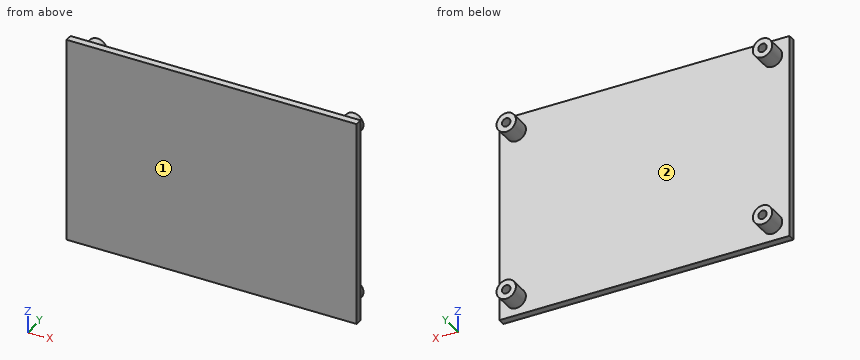
```python
from build123d import *

# Parameters (mm, degrees)
SKETCH1_W           = 120
SKETCH1_H           = 85
BOSS_EXTRUDE1_DEPTH = 3
SKETCH2_R           = 4
SKETCH2_R_2         = 1.75
BOSS_EXTRUDE2_DEPTH = 7.5


with BuildPart() as part:
    # Sketch1 → Boss-Extrude1 (new body)
    with BuildSketch(Plane(origin=(0, 0, 0), x_dir=(1, 0, 0), z_dir=(0, 1, 0))):
        with Locations((60, 42.5)):
            Rectangle(SKETCH1_W, SKETCH1_H)
    extrude(amount=BOSS_EXTRUDE1_DEPTH)

    # Sketch2 → Boss-Extrude2 (add)
    # profile 1 of 4: a face of its own
    with BuildSketch(Plane(origin=(0, 3, 0), x_dir=(1, 0, 0), z_dir=(0, 1, 0))):
        with Locations(Location((7, 78, 0), (0, 0, 90))):
            Circle(SKETCH2_R)
        with Locations(Location((7, 78, 0), (0, 0, 270))):
            Circle(SKETCH2_R_2, mode=Mode.SUBTRACT)
    # profile 2 of 4: a face of its own
    with BuildSketch(Plane(origin=(0, 3, 0), x_dir=(1, 0, 0), z_dir=(0, 1, 0))):
        with Locations(Location((7, 7, 0), (0, 0, 90))):
            Circle(SKETCH2_R)
        with Locations(Location((7, 7, 0), (0, 0, 270))):
            Circle(SKETCH2_R_2, mode=Mode.SUBTRACT)
    # profile 3 of 4: a face of its own
    with BuildSketch(Plane(origin=(0, 3, 0), x_dir=(1, 0, 0), z_dir=(0, 1, 0))):
        with Locations(Location((113, 7, 0), (0, 0, 90))):
            Circle(SKETCH2_R)
        with Locations(Location((113, 7, 0), (0, 0, 270))):
            Circle(SKETCH2_R_2, mode=Mode.SUBTRACT)
    # profile 4 of 4: a face of its own
    with BuildSketch(Plane(origin=(0, 3, 0), x_dir=(1, 0, 0), z_dir=(0, 1, 0))):
        with Locations(Location((113, 78, 0), (0, 0, 90))):
            Circle(SKETCH2_R)
        with Locations(Location((113, 78, 0), (0, 0, 270))):
            Circle(SKETCH2_R_2, mode=Mode.SUBTRACT)
    extrude(amount=BOSS_EXTRUDE2_DEPTH)


solid = part.part
```
Geometry check sheet. Reference: the model listing, model coordinates, mm. Face numbers are marked on the shaded views. A direction names the side the tool comes from. Coordinates: 2 decimals unless noted, no trailing zeros. Write each loop counter-clockwise with the first axis right and the second up, starting at its lowest first coordinate (ties: lowest second). Pieces come first, ordered by that corner, then holes. Notation, with made-up numbers: M 20,83 L 76,83 A25 cw 76,109 Z; hole C 76,32 d11. An arc over 180 degrees is marked long. One line per item, written item: value. Start each with the question number.
(1) Sectioned sample at C-C, the plane x = 7. Enter the section's corners in (y, z).
(2) Tool access check on the marked faces 1 and 2. Record the directions out of +Z, -Z, +X, -X, +Y, -Y that give a thin tool (end or side, any length) a straight path to the whole face; none if there is none.
(3) Sectioned sample at B-B, the plane z = -7. Enter the section's corners in (x, y), and give its area (4 significant figures).
(4) Sectioned sample at D-D, the plane z = -37.5. Enter the section's corners in (x, y), and give its area (3 significant figures).
(5) Depth check by flat-ended pin: pin 1 (1.5 mm diameter, centred on x = 45.5, z = -27.5, fed in from +Y). Enter the tip coordinate at first touch or a pass-through.
(6) Scan lines: line 1 along X through (y, z) = (6.5, -78); line 2 along Z through (x, y) = (113, 7.5); line 3 along Y through (x, z) = (65.5, -61). Record each from-to range of solid material in increasing order. Write a range as [from, to].
(7) Sectioned sample at A-A, the plane y = 4.5. Enter the section's corners in (x, z).
Filled sheet:
1. outline: M 0,-85 L 3,-85 L 3,-82 L 10.5,-82 L 10.5,-79.75 L 3,-79.75 L 3,-76.25 L 10.5,-76.25 L 10.5,-74 L 3,-74 L 3,-11 L 10.5,-11 L 10.5,-8.75 L 3,-8.75 L 3,-5.25 L 10.5,-5.25 L 10.5,-3 L 3,-3 L 3,0 L 0,0 Z
2. face 1: +Z, -Z, +X, -X, -Y
2. face 2: +Y
3. outline: M 0,0 L 120,0 L 120,3 L 117,3 L 117,10.5 L 114.75,10.5 L 114.75,3 L 111.25,3 L 111.25,10.5 L 109,10.5 L 109,3 L 11,3 L 11,10.5 L 8.75,10.5 L 8.75,3 L 5.25,3 L 5.25,10.5 L 3,10.5 L 3,3 L 0,3 Z
3. area: 427.5 mm²
4. outline: M 0,0 L 120,0 L 120,3 L 0,3 Z
4. area: 360 mm²
5. pin 1: y = 3
6. line 1: [3, 5.25], [8.75, 11], [109, 111.25], [114.75, 117]
6. line 2: [-82, -79.75], [-76.25, -74], [-11, -8.75], [-5.25, -3]
6. line 3: [0, 3]
7. outline: C 7,-78 d8; C 7,-7 d8; C 113,-78 d8; C 113,-7 d8; hole C 7,-78 d3.5; hole C 7,-7 d3.5; hole C 113,-78 d3.5; hole C 113,-7 d3.5
